```python
from build123d import *

# Parameters (mm, degrees)
F0_W     = 27.1145
F0_H     = 13.97
F0_W_2   = 22.0345
F0_H_2   = 7.46125
F1_DEPTH = 42.8625
F2_R     = 3.175
F3_R     = 4.03225
F4_DEPTH = 3.175
F6_DEPTH = 0.3175
F7_R     = 2.54


with BuildPart() as f1:
    # F0 (on Top) → F1 (new body, symmetric)
    with BuildSketch(Plane.XY):
        Rectangle(F0_W, F0_H)
        with Locations((0, 0.714375)):
            Rectangle(F0_W_2, F0_H_2, mode=Mode.SUBTRACT)
    extrude(amount=F1_DEPTH, both=True)

    # F2
    f2_edges = [f1.edges().sort_by_distance(p)[0] for p in [
        (13.55725, -6.985, 0),
        (-13.55725, -6.985, 0),
        (-13.55725, 6.985, 0),
        (13.55725, 6.985, 0),
        (-11.01725, 4.445, 0),
        (11.01725, 4.445, 0),
        (11.01725, -3.01625, 0),
        (-11.01725, -3.01625, 0),
    ]]
    fillet(f2_edges, radius=F2_R)

    # F3 (on face) → F4 (cut)
    with BuildSketch(Plane.XZ.offset(6.985)):
        with Locations((0, 26.9875)):
            Circle(F3_R)
    extrude(amount=-F4_DEPTH, mode=Mode.SUBTRACT)

    # F5 (on face) → F6 (join)
    with BuildSketch(Plane(origin=(0, 0, -42.8625), x_dir=(1, 0, 0), z_dir=(0, 0, -1))):
        with BuildLine():
            ThreePointArc((11.01725, -0.15875), (10.0873140303, 2.0863140303), (7.84225, 3.01625))
            Line((7.84225, 3.01625), (-7.84225, 3.01625))
            ThreePointArc((-7.84225, 3.01625), (-10.0873140303, 2.0863140303), (-11.01725, -0.15875))
            Line((-11.01725, -0.15875), (-11.01725, -1.27))
            ThreePointArc((-11.01725, -1.27), (-10.0873140303, -3.5150640303), (-7.84225, -4.445))
            Line((-7.84225, -4.445), (7.84225, -4.445))
            ThreePointArc((7.84225, -4.445), (10.0873140303, -3.5150640303), (11.01725, -1.27))
            Line((11.01725, -1.27), (11.01725, -0.15875))
        make_face()
    extrude(amount=-F6_DEPTH)

    # F7
    f7_edges = [f1.edges().sort_by_distance(p)[0] for p in [
        (0, -6.985, -42.8625),
        (12.627314, -6.055064, -42.8625),
        (13.55725, 0, -42.8625),
        (12.627314, 6.055064, -42.8625),
        (0, 6.985, -42.8625),
        (-12.627314, 6.055064, -42.8625),
        (-13.55725, 0, -42.8625),
        (-12.627314, -6.055064, -42.8625),
    ]]
    fillet(f7_edges, radius=F7_R)


solid = f1.part
```
Can you work these out from the model? Positions are in its coordinate system, mm. A direction names the side the tool comes from. Coordinates: 2 decimals unless noted, no trailing zeros. Write each loop counter-clockwise with the first axis right and the second up, starting at its lowest first coordinate (ties: lowest second). Pieces come first, ordered by that corner, then holes. Notation, with made-up numbers: M 48.5,-23.75 L 78.5,-23.75 A25 cw 78.5,15.25 Z; hole C 75.5,55 d10. An arc over 180 degrees is marked long. Write item = value, one per line. Start each with the question number.
Q1. Thinking about a two-plate mould opening in Y: for faces 4 (the face through (13.557, 0, 2)), 5 (the face through (-0.15, 6.22, -42.14)), 6 (the face through (-12.65, -6.03, 1.85)), 7 (the face through (0, 4.445, 1)), which applies, released by +Y, released by -Y, zero draft, split by the parting line, or undercut?
Q2. If we section it at B-B, the plane x = 0: Write out the boundary of the cut face in (y, z) (1 decimal).
Q3. If we section it at C-C, the plane y = 2.5: Write out the boundary of the cut face in (x, z) (1 decimal), then the cut area to 3 significant figures.
Q4. If we section it at A-A, the plane z = -3: Write out the boundary of the cut face in (x, y) (3 decimals).
Q5. I'm going to push flat-ended pins straight in: pin 1 (2 mm diameter, centred on x = -3, y = 1.5, fed in from +Z) (3 decimals); pin 2 (4 mm diameter, centred on x = 0.5, z = 27.5, fed in from -Y). Where does each tip first touch, or does it pass through?
Q6. If I drill on L1, parallel to Y at x = 5.75, z = -3 (3 decimals); L2, parallel to X at y = 0.25, z = -10; L3, parallel to Z at x = 0, y = -5.35, over which ranges is the centre line in solid material (lowest first)? Write a range as [from, to].
Q7. On a 3-axis mill with a long thin cutter (end or side, diameter ignored), from which of +Z, -Z, +X, -X, +Y, -Y can I reach the whole of each face in a straight line? I mean faces 1 (the face through (0, -3.81, 27)), 2 (the face through (10.112, -2.061, -0.439)), 3 (the face through (12.65, -6.03, 1.85)). Say none if no direction works.
Q8. If we section it at D-D, the plane x = 7: Write out the boundary of the cut face in (y, z) (1 decimal), then the cut area to 3 significant figures.
Check sheet entries:
q1.face_4 = zero draft
q1.face_5 = released by +Y
q1.face_6 = released by -Y
q1.face_7 = undercut
q2.outline = M -7,-40.3 A2.5 ccw -4.4,-42.9 L 4.4,-42.9 A2.5 ccw 7,-40.3 L 7,42.9 L 4.4,42.9 L 4.4,-42.5 L -3,-42.5 L -3,42.9 L -7,42.9 L -7,31 L -3.8,31 L -3.8,23 L -7,23 Z
q3.outline = M -13.6,-40.3 A2.5 ccw -11,-42.9 L 11,-42.9 A2.5 ccw 13.6,-40.3 L 13.6,42.9 L 10.8,42.9 L 10.8,-42.5 L -10.8,-42.5 L -10.8,42.9 L -13.6,42.9 Z
q3.area = 482 mm²
q4.outline = M -13.557,-3.81 A3.175 ccw -10.382,-6.985 L 10.382,-6.985 A3.175 ccw 13.557,-3.81 L 13.557,3.81 A3.175 ccw 10.382,6.985 L -10.382,6.985 A3.175 ccw -13.557,3.81 Z; hole M -11.017,0.159 A3.175 ccw -7.842,-3.016 L 7.842,-3.016 A3.175 ccw 11.017,0.159 L 11.017,1.27 A3.175 ccw 7.842,4.445 L -7.842,4.445 A3.175 ccw -11.017,1.27 Z
q5.pin_1 = -42.545
q5.pin_2 = -3.81
q6.L1 = [-6.985, -3.016], [4.445, 6.985]
q6.L2 = [-13.56, -11.02], [11.02, 13.56]
q6.L3 = [-42.7, 22.96], [31.02, 42.86]
q7.face_1 = -Y
q7.face_2 = +Z
q7.face_3 = +Z, -Z, +X, -Y
q8.outline = M -7,-40.3 A2.5 ccw -4.4,-42.9 L 4.4,-42.9 A2.5 ccw 7,-40.3 L 7,42.9 L 4.4,42.9 L 4.4,-42.5 L -3,-42.5 L -3,42.9 L -7,42.9 Z
q8.area = 558 mm²
